Autodesk Inventor part; units mm, degrees
ref_plane "YZ Plane" through (0, 0, 0) normal (1, 0, 0) x (0, 1, 0)
ref_plane "XZ Plane" through (0, 0, 0) normal (0, 1, 0) x (-1, 0, 0)
ref_plane "XY Plane" through (0, 0, 0) normal (0, 0, 1) x (1, 0, 0)
sketch "Sketch1" plane through (0, 0, 0) normal (0, 1, 0) x (-1, 0, 0)
  line L0 (0, 0) -> (43, 0)
  line L1 (43, 0) -> (43, -61)
  line L2 (43, -61) -> (0, -61)
  line L3 (0, -61) -> (0, 0)
  dimension "d0" = 61
  dimension "d1" = 43
extrude "Extrusion1" add sketch "Sketch1" along normal blind 10
sketch "Sketch2" plane through (0, 0, 0) normal (1, 0, 0) x (0, 0, -1)
  line L0 (0, 0) -> (0, 10)
  line L1 (0, 5) -> (12.5, 5)
  circle A0 centre (12.5, 5) radius 1.25
  line L2 (0, 10) -> (61, 10)
  line L3 (30.5, 10) -> (30.5, 0)
  circle A1 centre (48.5, 5) radius 1.25
  dimension "d4" = 12.5
  dimension "d5" = 2.5
extrude "Extrusion2" cut sketch "Sketch2" against normal blind 5
sketch "Sketch3" plane through (-43, 0, -61) normal (-1, 0, 0) x (0, 0, 1)
  line L0 (61, 0) -> (0, 0)
  line L1 (61, 0) -> (61, 10)
  line L2 (0, 10) -> (61, 10)
  line L3 (0, 0) -> (0, 10)
  circle A0 centre (48.5, 5) radius 1.25
  circle A1 centre (12.5, 5) radius 1.25
extrude "Extrusion3" cut sketch "Sketch3" against normal blind 5 contours A0 | A1
sketch "Sketch4" plane through (0, 10, 0) normal (0, 1, 0) x (1, 0, 0)
  line L0 (-43, 0) -> (0, 0)
  line L1 (0, 61) -> (-43, 61)
  line L2 (-21.5, 0) -> (-21.5, 6.35)
  line L3 (-21.5, 61) -> (-21.5, 54.65)
  circle A0 centre (-21.5, 6.35) radius 1.25
  circle A1 centre (-21.5, 54.65) radius 1.25
  dimension "d10" = 6.35
  dimension "d11" = 6.35
  dimension "d12" = 2.5
  dimension "d13" = 2.5
extrude "Extrusion4" cut sketch "Sketch4" against normal up to surface (10 mm away)
sketch "Sketch5" plane through (0, 10, 0) normal (0, 1, 0) x (1, 0, 0)
  circle A0 centre (-21.5, 6.35) radius 1.25
  circle A1 centre (-21.5, 54.65) radius 1.25
  line L0 (-43, 0) -> (0, 0)
  line L1 (0, 0) -> (0, 61)
  line L2 (0, 61) -> (-43, 61)
  line L3 (-43, 61) -> (-43, 0)
  line L4 (-8.8, 11.45) -> (-34.2, 11.45)
  line L5 (-34.2, 11.45) -> (-34.2, 49.55)
  line L6 (-34.2, 49.55) -> (-8.8, 49.55)
  line L7 (-8.8, 49.55) -> (-8.8, 11.45)
  line L8 (-8.8, 11.45) -> (-34.2, 49.55) construction
  line L9 (-34.2, 11.45) -> (-8.8, 49.55) construction
  point P0 (-21.5, 30.5)
  dimension "d16" = 25.4
  dimension "d17" = 38.1
extrude "Extrusion5" cut sketch "Sketch5" against normal up to surface (10 mm away) contours L4 L5 L6 L7
properties part number "bottomTiltOnly"
Can you work these out from the model? Positions are in its coordinate system, mm. A direction names the side the tool comes from. Coordinates: 2 decimals unless noted, no trailing zeros. Loops run counter-clockwise (first coordinate to the right, second up) from the corner with the lowest first, then second, coordinate; pieces in that order, holes last.
Item 1: I'm going to push flat-ended pins straight in: pin 1 (2 mm diameter, centred on y = 5, z = -12.5, fed in from +X); pin 2 (2 mm diameter, centred on y = 3.5, z = -43.5, fed in from +X); pin 3 (0.8 mm diameter, centred on y = 4.5, z = -12.5, fed in from -X); pin 4 (1.5 mm diameter, centred on x = -21.5, z = -6.35, fed in from -Y). Where does each tip first touch, or does it pass through?
Answers below:
pin 1: stops at x = -5
pin 2: stops at x = 0
pin 3: stops at x = -38
pin 4: passes through
Item 2: Suppose I cut it at C-C (y = 5). Please give me the cut outline in (x, z).
Answers below:
outline: (-43, -61) - (0, -61) - (0, -49.75) - (-5, -49.75) - (-5, -47.25) - (0, -47.25) - (0, -13.75) - (-5, -13.75) - (-5, -11.25) - (0, -11.25) - (0, 0) - (-43, 0) - (-43, -11.25) - (-38, -11.25) - (-38, -13.75) - (-43, -13.75) - (-43, -47.25) - (-38, -47.25) - (-38, -49.75) - (-43, -49.75) - close; hole (-34.2, -49.55) - (-8.8, -49.55) - (-8.8, -11.45) - (-34.2, -11.45) - close; hole circle Ø2.5 at (-21.5, -54.65); hole circle Ø2.5 at (-21.5, -6.35)
Item 3: Please list where these lines run through material, in increasing order: L1, parallel to X at y = 2.75, z = -37.5; L2, parallel to Z at x = -9.5, y = 1.5; L3, parallel to Y at x = -41.7, z = -48.5.
Answers below:
L1: x = -43 to -34.2, -8.8 to 0
L2: z = -61 to -49.55, -11.45 to 0
L3: y = 0 to 3.75, 6.25 to 10
Item 4: If we mould it in two halves opening along X, with no side actions, what happens to faces 1 (the face through (-5, 5, -12)), 2 (the face through (-36, 10, -30)), 3 (the face through (-34.2, 5, -30))? For each: released by +X, released by -X, zero draft, split by the parting line, or undercut.
Answers below:
face 1: released by +X
face 2: zero draft
face 3: undercut
Item 5: Suppose I cut it at A-A (z = -54.65). Please give me the cut outline in (x, y), then the cut area to 3 significant figures.
Answers below:
outline: (-43, 0) - (-22.75, 0) - (-22.75, 10) - (-43, 10) - close; (-20.25, 0) - (0, 0) - (0, 10) - (-20.25, 10) - close
area: 405 mm2
Item 6: Which directions (+Z, -Z, +X, -X, +Y, -Y) give clear straight access to the entire face, cutting with the end or side of a thin tool? Please do faces 4 (the face through (-21, 5, -11.45)), 5 (the face through (-2.46, 4.24, -47.51)), 6 (the face through (0, 5, -31)), 7 (the face through (-40.53, 4.24, -13.49)).
Answers below:
face 4: +Y, -Y
face 5: +X
face 6: +Z, -Z, +X, +Y, -Y
face 7: -X
Item 7: Suppose I cut it at D-D (x = -3). Please give me the cut outline in (y, z), then the cut area to 3 significant figures.
Answers below:
outline: (0, -61) - (10, -61) - (10, 0) - (0, 0) - close; hole circle Ø2.5 at (5, -48.5); hole circle Ø2.5 at (5, -12.5)
area: 600 mm2
Item 8: Suppose I cut it at B-B (x = -24.5). Please give me the cut outline in (y, z).
Answers below:
outline: (0, -61) - (10, -61) - (10, -49.55) - (0, -49.55) - close; (0, -11.45) - (10, -11.45) - (10, 0) - (0, 0) - close
